from build123d import *

# Parameters (mm, degrees)
F1_DEPTH = 25.4
F2_R     = 12.69999
F3_R     = 6.35
F4_DEPTH = 25.4
F6_DEPTH = 25.4


# Not quite as in the source:
# - a fillet or chamfer is up to 0.001 mm smaller than in the source, because OpenCascade refuses the exact size


with BuildPart() as f1:
    # F0 (on Front) → F1 (new body)
    with BuildSketch(Plane.XZ):
        Polygon((0, 38.1), (0, 0), (76.2, 0), (76.2, 12.7), (25.4, 12.7), (25.4, 38.1), align=None)
    extrude(amount=F1_DEPTH)

    # F2 (radius 12.7 in the source; OpenCascade refuses exactly that, so slightly less here)
    f2_edges = [f1.edges().sort_by_distance(p)[0] for p in [
        (25.4, -12.7, 38.1),
        (0, -12.7, 38.1),
        (76.2, -25.4, 6.35),
        (76.2, 0, 6.35),
    ]]
    fillet(f2_edges, radius=F2_R)

    # F3 (on face) → F4 (cut)
    with BuildSketch(Plane.XZ.offset(25.4)):
        with Locations((12.7, 25.4)):
            Circle(F3_R)
    extrude(amount=-F4_DEPTH, mode=Mode.SUBTRACT)

    # F5 (on face) → F6 (cut)
    with BuildSketch(Plane.XY.offset(12.7)):
        with BuildLine():
            ThreePointArc((44.45, -19.05), (48.9401287414, -17.1901284329), (50.8000010533, -12.7))
            ThreePointArc((50.8000010533, -12.7), (48.9401287414, -8.2098715671), (44.45, -6.35))
            ThreePointArc((44.45, -6.35), (38.1000010533, -12.7), (44.45, -19.05))
        make_face()
        with BuildLine():
            ThreePointArc((44.45, -6.35), (48.9401287414, -8.2098715671), (50.8000010533, -12.7))
            ThreePointArc((50.8000010533, -12.7), (48.9401287414, -17.1901284329), (44.45, -19.05))
            Line((44.45, -19.05), (63.5, -19.05))
            ThreePointArc((63.5, -19.05), (57.15, -12.7), (63.5, -6.35))
            Line((63.5, -6.35), (44.45, -6.35))
        make_face()
        with BuildLine():
            ThreePointArc((69.85, -12.7), (67.9901280605, -8.2098719395), (63.5, -6.35))
            ThreePointArc((63.5, -6.35), (57.15, -12.7), (63.5, -19.05))
            ThreePointArc((63.5, -19.05), (67.9901280605, -17.1901280605), (69.85, -12.7))
        make_face()
    extrude(amount=-F6_DEPTH, mode=Mode.SUBTRACT)


solid = f1.part
Read the model definition and answer for the solid it produces. Units are mm, in the model's axes. A direction names the side the tool comes from. Give positions to 0.01 mm unless a question says otherwise; leave off trailing zeros. Loops run counter-clockwise (first coordinate to the right, second up) from the corner with the lowest first, then second, coordinate; pieces in that order, holes last. Notation, with made-up numbers: (-10, 45) - (9, 45) arc R12 ccw to (9, 54) - close; hole circle Ø6 at (-30, 42.5). An arc over 180 degrees is marked (long way). Answer as CSV lines item,"result". Start each with the question number.
1) Which of the six approach directions +Z, -Z, +X, -X, +Y, -Y give full straight-line access (tool end or side, diameter ignored) to faces 1 (the face through (25.4, -13, 19)), 2 (the face through (54, -6.35, 6)), 3 (the face through (72.58, -21.58, 6.44))?
2) Find section A-A (x = 52). Write down the section's boundary in (y, z).
3) Straight lines are drawn through the part: L1, parallel to Z at x = 12.7, y = -14.75; L2, parallel to Y at x = 45.5, z = 2.5; L3, parallel to X at y = -5.25, z = 17.5. For each, find the intervals that lie inside material, in ascending order. Write a range as from..to.
4) Each of these flat-tipped pins is pushed along its axis until it touches: pin 1 Ø1.5 at (x, y) = (14, -10) entering from +Z; pin 2 Ø10 at (y, z) = (-11.5, 33) entering from +X; pin 3 Ø4 at (y, z) = (-7, 21.5) entering from +X. Where does it stop, or does it pass through?
5) Find section B-B (y = -16.5). State how many separate pieces and enclosed holes the cut face has, then the cut area to 3 significant figures.
6) Determine the mould class of faces 4 (the face through (24, 0, 15)), 5 (the face through (29, -13, 0)), 6 (the face through (46, -21, 12.7)), 7 (the face through (7.66, -12.88, 21.54)) for opening direction Z: released by +Z, released by -Z, zero draft, split by the parting line, or undercut.
Findings below:
1,face 1,"+Z, +X, +Y, -Y"
1,face 2,"+Z, -Z"
1,face 3,"+Z, -Z, +X, -Y"
2,outline,"(-25.4, 0) - (-19.05, 0) - (-19.05, 12.7) - (-25.4, 12.7) - close; (-6.35, 0) - (0, 0) - (0, 12.7) - (-6.35, 12.7) - close"
3,L1,"0..19.05, 31.75..38.1"
3,L2,"-25.4..-19.05, -6.35..0"
3,L3,"0..25.4"
4,pin 1,"z = 38.09"
4,pin 2,"x = 25.13"
4,pin 3,"x = 25.4"
5,separate pieces,"2"
5,enclosed holes,"1"
5,area,"1,040 mm^2"
6,face 4,"zero draft"
6,face 5,"released by -Z"
6,face 6,"released by +Z"
6,face 7,"undercut"
